The drawing under review shows one solid part. Ordinate dimensions are in mm from its lowest x, y, z. A direction names the side the tool comes from. Round coordinates to 2 decimals unless told otherwise and drop trailing zeros. Write each loop counter-clockwise with the first axis right and the second up, starting at its lowest first coordinate (ties: lowest second). Pieces come first, ordered by that corner, then holes. Notation, with made-up numbers: M -1.5,46.5 L 52.5,46.5 A21 cw 52.5,64.5 Z; hole C 34,26 d11. An arc over 180 degrees is marked long. One line per item, written item: value. Start each with the question number.
1) For P1, Ø1, axis at x = 10.5, z = 30, coming from the -Y side, flat-tipped, find the tip position at first contact; note if it passes through.
2) Tool access review of the marked faces 1 and 2: name each direction out of +Z, -Z, +X, -X, +Y, -Y from which nothing blocks a thin tool from reaching the whole face with its end or side.
3) Take a section at C-C, the plane y = 3. Write out the cut boundary in (x, z) (1 decimal).
4) Take a section at D-D, the plane y = 18. Write out the cut boundary in (x, z).
5) Take a section at A-A, the plane x = 12.25. Write out the cut boundary in (y, z), and give its area (3 significant figures).
6) Wall thickness on probe 1 along Y at (x, z) = (7.5, 177) (1 decimal); probe 2 along X at (y, z) = (6.5, 65); probe 3 along Z at (x, y) = (3.5, 21): over which ranges is each line inside the solid? List them lowest first.
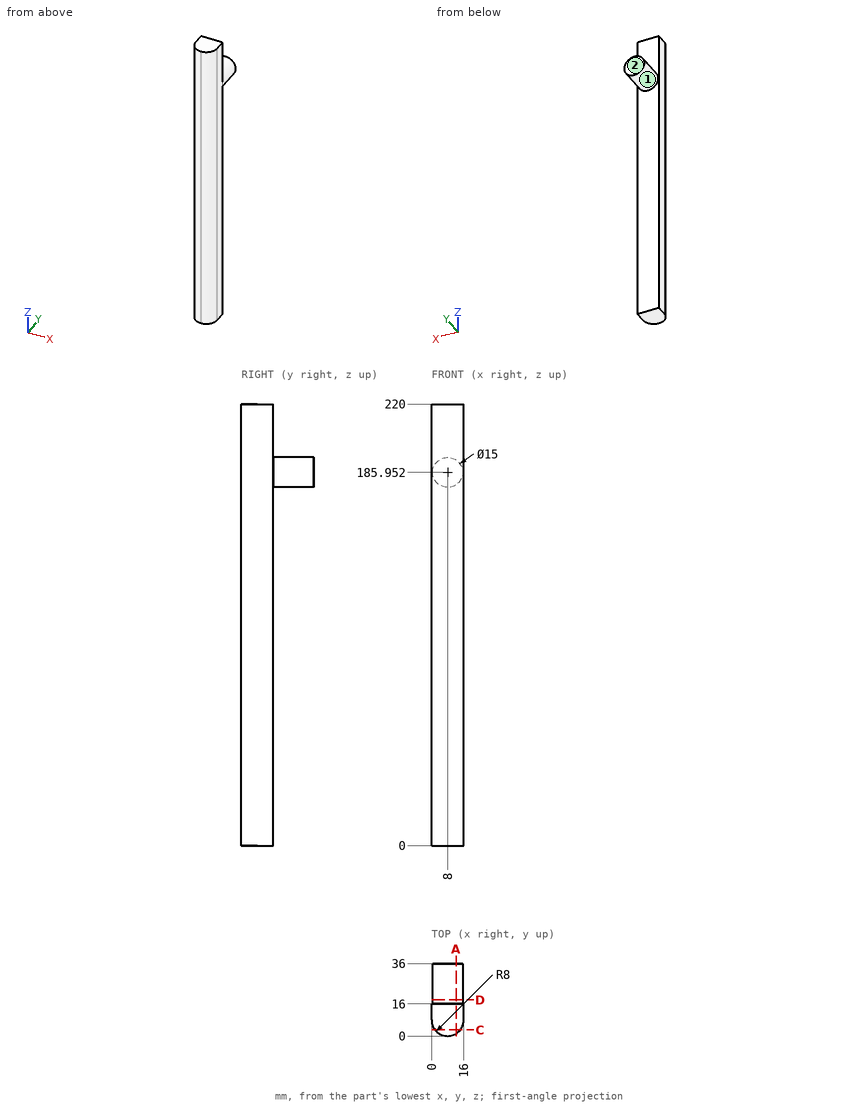
Checked values:
1. P1: stops at y = 0.25
2. face 1: +Y
2. face 2: +Z, -Z, +X, -X, +Y
3. outline: M 1.8,0 L 14.2,0 L 14.2,220 L 1.8,220 Z
4. outline: C 8,185.95 d15
5. outline: M 1.22,0 L 16,0 L 16,179.77 L 36,179.77 L 36,192.13 L 16,192.13 L 16,220 L 1.22,220 Z
5. area: 3,500 mm2
6. probe 1: y = 0 to 16
6. probe 2: x = 0.14 to 15.86
6. probe 3: z = 179.95 to 191.95
